Print and shaded views of the part. All mm, measured from the part's lowest x, y and z. A direction names the side the tool comes from. Coordinates: 2 decimals unless noted, no trailing zeros. Order: outer loops, then holes, each group sorted by start corner. A loop starts at its lowest first (then second) coordinate and runs counter-clockwise, first axis right, second up.
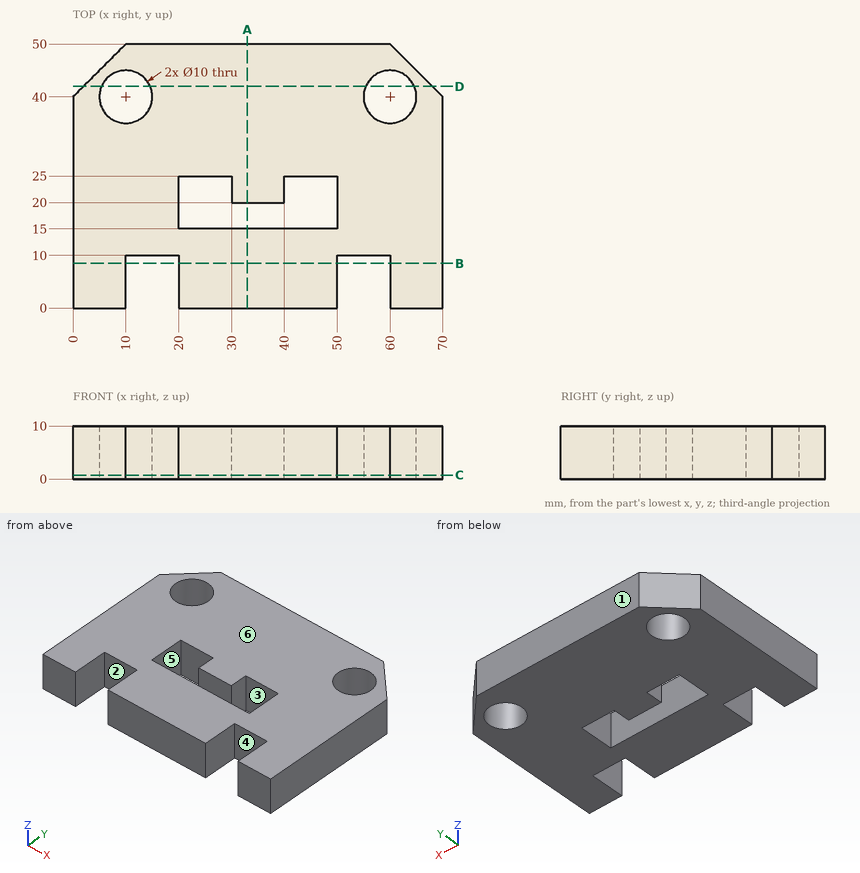
Q1. Cut at C-C, the plane z = 0.75. List the corners of the cut face in (x, y), plus the area to 3 significant figures.
Established:
outline: (0, 0) - (10, 0) - (10, 10) - (20, 10) - (20, 0) - (50, 0) - (50, 10) - (60, 10) - (60, 0) - (70, 0) - (70, 40) - (60, 50) - (10, 50) - (0, 40) - close; hole circle Ø10 at (10, 40); hole (20, 15) - (50, 15) - (50, 25) - (40, 25) - (40, 20) - (30, 20) - (30, 25) - (20, 25) - close; hole circle Ø10 at (60, 40)
area: 2,790 mm2
Q2. Drop a flat-ended pin along its axis: P1, Ø3, axis at x = 17.5, z = 3.5, coming from the -Y side. Give the stop position or say it passes through.
Established:
P1: stops at y = 10
Q3. Cut at B-B, the plane y = 8.5. List the corners of the cut face in (x, z), plus the area to 3 significant figures.
Established:
outline: (0, 0) - (10, 0) - (10, 10) - (0, 10) - close; (20, 0) - (50, 0) - (50, 10) - (20, 10) - close; (60, 0) - (70, 0) - (70, 10) - (60, 10) - close
area: 500 mm2
Q4. Mould opens along Y. For the marked faces 4, 5 and 6 say: pulls with the +Y half, pulls with the -Y half, needs draft (parallel to the pull), parting line crosses it, or undercut.
Established:
face 4: pulls with the -Y half
face 5: undercut
face 6: needs draft
Q5. Which spindle directions (+Z, -Z, +X, -X, +Y, -Y) get a long thin tool onto all of the face, cutting with end or side? Do the marked faces 1, 2 and 3. Say none if no direction does.
Established:
face 1: +Z, -Z, +X, -X, +Y
face 2: +Z, -Z, -Y
face 3: +Z, -Z
Q6. Cut at D-D, the plane y = 42. List the corners of the cut face in (x, z), plus the area to 3 significant figures.
Established:
outline: (2, 0) - (5.42, 0) - (5.42, 10) - (2, 10) - close; (14.58, 0) - (55.42, 0) - (55.42, 10) - (14.58, 10) - close; (64.58, 0) - (68, 0) - (68, 10) - (64.58, 10) - close
area: 477 mm2
Q7. Probe line 1 (X direction, y = 3, z = 7.5); line 2 (Y direction, x = 22, z = 3.25); line 3 (X direction, y = 43, z = 4.5). List the from-to ranges inside material, lowest first.
Established:
line 1: x = 0 to 10, 20 to 50, 60 to 70
line 2: y = 0 to 15, 25 to 50
line 3: x = 3 to 6, 14 to 56, 64 to 67
Q8. Cut at A-A, the plane x = 33. List the corners of the cut face in (y, z), plus the area to 3 significant figures.
Established:
outline: (0, 0) - (15, 0) - (15, 10) - (0, 10) - close; (20, 0) - (50, 0) - (50, 10) - (20, 10) - close
area: 450 mm2
